Print and shaded views of the part. All mm, measured from the part's lowest x, y and z. A direction names the side the tool comes from. Round coordinates to 2 decimals unless told otherwise and drop trailing zeros. Order: outer loops, then holes, each group sorted by start corner. A loop starts at its lowest first (then second) coordinate and runs counter-clockwise, first axis right, second up. Notation, with made-up numbers: (48, -17) - (58, -17) arc R27 ccw to (58, 8) - close; hole circle Ø3 at (38.25, 28.25). An arc over 180 degrees is marked (long way). Return JSON: item names as keys, results as strings. Group by question number.
Item 1: Probe probe 1 along X at (y, z) = (76.5, 11.5); probe 2 along Y at (x, z) = (20.5, 17.5); probe 3 along Y at (x, z) = (5.5, 12.25). List the from-to ranges inside material, lowest first.
Item 2: Saw through at A-A on z = 12. List the corners of the cut face in (x, y).
Item 3: Drop flat-ended pins along their axis: pin 1 (1.5 mm diameter, centred on x = 13.5, y = 47.5, fed in from -Z); pin 2 (4 mm diameter, centred on y = 92, z = 7.5, fed in from +X); pin 3 (2 mm diameter, centred on x = 16, y = 70.5, fed in from -Z). Give the stop position or say it passes through.
Item 4: Saw through at C-C on y = 67.5. List the corners of the cut face in (x, z).
Item 5: Saw through at D-D on x = 20.75. List the corners of the cut face in (y, z), and give its area (3 significant figures).
Item 6: Tool access for the marked faces 1 and 2: list every direction of +Z, -Z, +X, -X, +Y, -Y with a clear straight run to the whole face (end or side of a thin tool).
Item 7: Saw through at B-B on x = 12. List the corners of the cut face in (y, z).
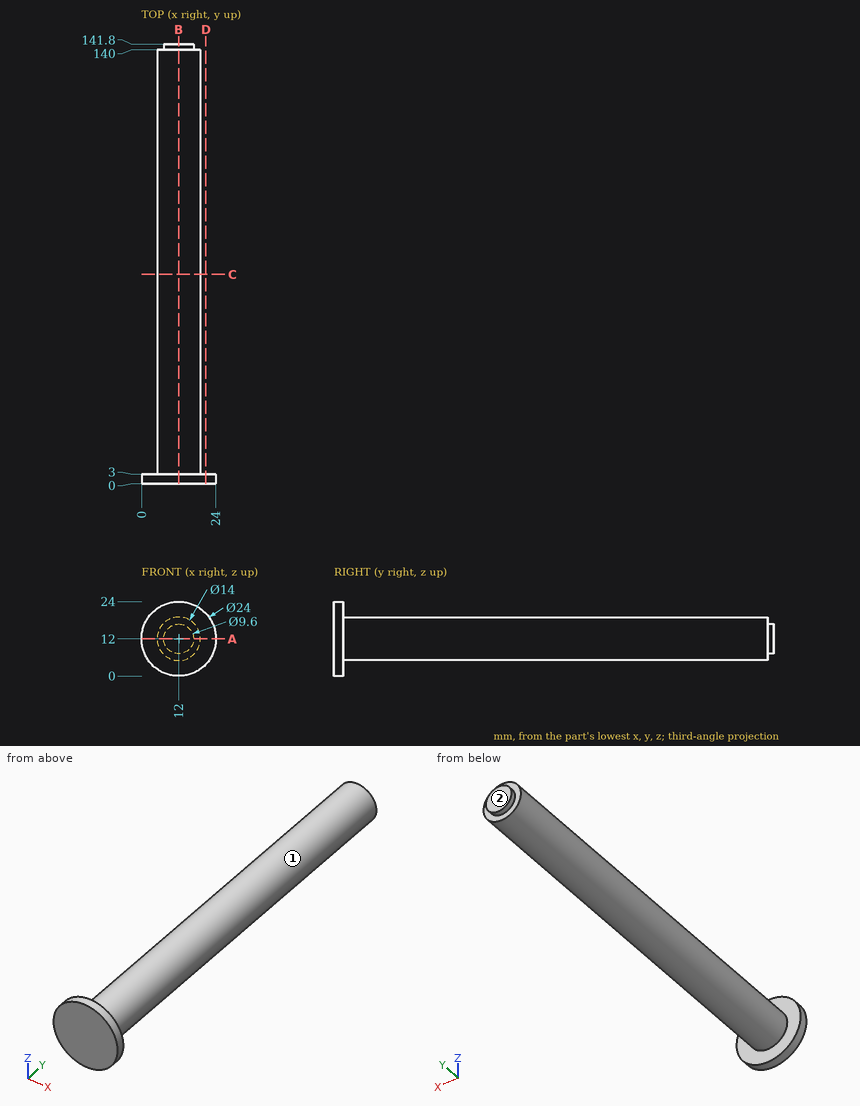
Filled in:
{
 "1": {"probe 1": "x = 5.02 to 18.98", "probe 2": "y = 0 to 3", "probe 3": "y = 0 to 140"},
 "2": {"outline": "(0, 0) - (24, 0) - (24, 3) - (19, 3) - (19, 140) - (16.8, 140) - (16.8, 141.8) - (7.2, 141.8) - (7.2, 140) - (5, 140) - (5, 3) - (0, 3) - close"},
 "3": {"pin 1": "stops at z = 5.04", "pin 2": "stops at x = 18.54", "pin 3": "stops at z = 5.68"},
 "4": {"outline": "circle Ø14 at (12, 12)"},
 "5": {"outline": "(0, 3.79) - (3, 3.79) - (3, 20.21) - (0, 20.21) - close", "area": "49.3 mm^2"},
 "6": {"face 1": "+Y", "face 2": "+Z, -Z, +X, -X, +Y"},
 "7": {"outline": "(0, 0) - (3, 0) - (3, 5) - (140, 5) - (140, 7.2) - (141.8, 7.2) - (141.8, 16.8) - (140, 16.8) - (140, 19) - (3, 19) - (3, 24) - (0, 24) - close"}
}
